```python
from build123d import *

# Parameters (mm, degrees)
SKETCH1_R               = 11
BOSS_EXTRUDE1_DEPTH     = 1.6
SKETCH2_R               = 8
BOSS_EXTRUDE2_DEPTH     = 9.5
SKETCH3_R               = 11
BOSS_EXTRUDE3_DEPTH     = 1.6
CUT_EXTRUDE1_DEPTH      = 21.082081565
CUT_EXTRUDE1_DEPTH_BACK = 21.082081565
SKETCH4_R               = 4


with BuildPart() as part:
    # Sketch1 → Boss-Extrude1 (new body)
    with BuildSketch(Plane(origin=(0, 0, 0), x_dir=(1, 0, 0), z_dir=(0, 1, 0))):
        with Locations(Location((0, 0, 0), (0, 0, 270))):
            Circle(SKETCH1_R)
    extrude(amount=BOSS_EXTRUDE1_DEPTH)

    # Sketch2 → Boss-Extrude2 (add)
    with BuildSketch(Plane(origin=(0, 1.6, 0), x_dir=(1, 0, 0), z_dir=(0, 1, 0))):
        with Locations(Location((0, 0, 0), (0, 0, 270))):
            Circle(SKETCH2_R)
    extrude(amount=BOSS_EXTRUDE2_DEPTH)

    # Sketch3 → Boss-Extrude3 (add)
    with BuildSketch(Plane(origin=(0, 11.1, 0), x_dir=(1, 0, 0), z_dir=(0, 1, 0))):
        with Locations(Location((0, 0, 0), (0, 0, 270))):
            Circle(SKETCH3_R)
    extrude(amount=BOSS_EXTRUDE3_DEPTH)

    # Sketch4 → Cut-Extrude1 (cut, two sides: drawn at the far end of the back side and taken through both)
    with BuildSketch(Plane(origin=(0, 12.7, 0), x_dir=(1, 0, 0), z_dir=(0, 1, 0)).offset(-CUT_EXTRUDE1_DEPTH_BACK)):
        with Locations(Location((0, 0, 0), (0, 0, 270))):
            Circle(SKETCH4_R)
    extrude(amount=CUT_EXTRUDE1_DEPTH + CUT_EXTRUDE1_DEPTH_BACK, mode=Mode.SUBTRACT)


solid = part.part
```
Part model, mm, in its own coordinate system. A direction names the side the tool comes from. Coordinates: 2 decimals unless noted, no trailing zeros. Loops run counter-clockwise (first coordinate to the right, second up) from the corner with the lowest first, then second, coordinate; pieces in that order, holes last. Notation, with made-up numbers: (36.5, -18) - (62.5, -18) arc R27 ccw to (62.5, 16) - close; hole circle Ø4 at (36.5, -11.75). An arc over 180 degrees is marked (long way). Write item = value, one per line. Start each with the question number.
Item 1: Flat gauge pins, fed straight in: pin 1 Ø6 at (x, y) = (2, 4.5) entering from -Z; pin 2 Ø6.5 at (x, z) = (1.5, 0.5) entering from +Y; pin 3 Ø5 at (x, y) = (-1.5, 9) entering from +Z. Where does each tip first touch, or does it go through?
Item 2: 3-axis set-ups, long thin cutter, end or side, ignore diameter. For faces 1 (the flat face through (-8, 1.6, -2)), 2 (the flat face through (-5, 0, 0)): which of +Z, -Z, +X, -X, +Y, -Y reach the whole face in a straight line?
Item 3: Wall check: L1, parallel to X at y = 6.5, z = 0; L2, parallel to Y at x = 4.75, z = 9; L3, parallel to Z at x = -3.25, y = 6.5. Give the ranges that are in metal, low to high. Write a range as from..to.
Item 4: Mould opens along Z. For faces 3 (the cylindrical face through (-10.74, 11.89, -2.38)), 4 (the flat face through (-8, 11.1, -2)), 5 (the cylindrical face through (-3.905, 6.261, -0.867)) say: released by +Z, released by -Z, zero draft, split by the parting line, or undercut.
Item 5: Cut at C-C, the plane z = 7.5. Give the cut face in (x, y).
Item 6: Cut at B-B, the plane x = 0. Give the cut face in (y, z).
Item 7: Cut at A-A, the plane z = 0. Give the cut face in (x, y), and give its area (3 significant figures).
Item 8: Cut at D-D, the plane y = 6. Give the cut face in (x, z), and give its area (3 significant figures).
The answers:
q1.pin_1 = -10.93
q1.pin_2 = 12.7
q1.pin_3 = 11
q2.face_1 = none
q2.face_2 = +Z, -Z, +X, -X, -Y
q3.L1 = -8..-4, 4..8
q3.L2 = 0..1.6, 11.1..12.7
q3.L3 = -7.31..-2.33, 2.33..7.31
q4.face_3 = split by the parting line
q4.face_4 = zero draft
q4.face_5 = undercut
q5.outline = (-8.05, 0) - (8.05, 0) - (8.05, 1.6) - (2.78, 1.6) - (2.78, 11.1) - (8.05, 11.1) - (8.05, 12.7) - (-8.05, 12.7) - (-8.05, 11.1) - (-2.78, 11.1) - (-2.78, 1.6) - (-8.05, 1.6) - close
q6.outline = (0, -11) - (1.6, -11) - (1.6, -8) - (11.1, -8) - (11.1, -11) - (12.7, -11) - (12.7, -4) - (0, -4) - close; (0, 4) - (12.7, 4) - (12.7, 11) - (11.1, 11) - (11.1, 8) - (1.6, 8) - (1.6, 11) - (0, 11) - close
q7.outline = (-11, 0) - (-4, 0) - (-4, 12.7) - (-11, 12.7) - (-11, 11.1) - (-8, 11.1) - (-8, 1.6) - (-11, 1.6) - close; (4, 0) - (11, 0) - (11, 1.6) - (8, 1.6) - (8, 11.1) - (11, 11.1) - (11, 12.7) - (4, 12.7) - close
q7.area = 121 mm2
q8.outline = circle Ø16 at (0, 0); hole circle Ø8 at (0, 0)
q8.area = 151 mm2
